Geometry: final body of the model. Coordinates: model frame, mm. Face numbers are marked on the shaded views. Give positions to 0.01 mm unless a question says otherwise; leave off trailing zeros. Order: outer loops, then holes, each group sorted by start corner. A loop starts at its lowest first (then second) coordinate and runs counter-clockwise, first axis right, second up. Notation, with made-up numbers: (81.25, 1.25) - (132.25, 1.25) arc R33 cw to (132.25, 31.25) - close; hole circle Ø1 at (76.5, -34). An arc over 180 degrees is marked (long way). One line per item, written item: value.
```python
from build123d import *

# Parameters (mm, degrees)
SKETCH1_R                 = 3
BOSS_EXTRUDE1_DEPTH       = 24
CHAMFER1_SIZE             = 1
M4X0_7_TAPPED_HOLE1_D     = 3.3
M4X0_7_TAPPED_HOLE1_DEPTH = 6
M4X0_7_TAPPED_HOLE1_TIP   = 0.991420021


with BuildPart() as part:
    # Sketch1 → Boss-Extrude1 (new body)
    with BuildSketch(Plane(origin=(0, 0, 0), x_dir=(1, 0, 0), z_dir=(0, 1, 0))):
        with Locations(Location((0, 0, 0), (0, 0, 270))):
            Circle(SKETCH1_R)
    extrude(amount=BOSS_EXTRUDE1_DEPTH)

    # Chamfer1
    chamfer1_edges = [part.edges().sort_by_distance(p)[0] for p in [
        (0, 24, -3),
    ]]
    chamfer(chamfer1_edges, length=CHAMFER1_SIZE)

    # M4x0.7 Tapped Hole1
    with Locations(Plane.XZ):
        with Locations((0, 0)):
            Hole(M4X0_7_TAPPED_HOLE1_D / 2, depth=M4X0_7_TAPPED_HOLE1_DEPTH)
            with Locations((0, 0, -(M4X0_7_TAPPED_HOLE1_DEPTH + M4X0_7_TAPPED_HOLE1_TIP / 2))):  # 118° drill point
                Cone(0, M4X0_7_TAPPED_HOLE1_D / 2, M4X0_7_TAPPED_HOLE1_TIP, mode=Mode.SUBTRACT)


solid = part.part
```
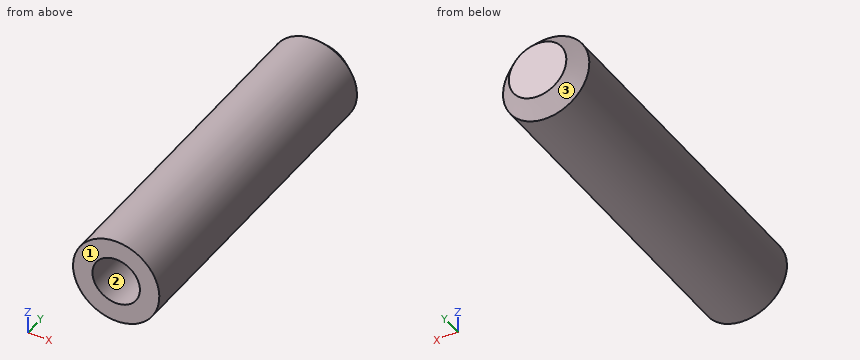
1) Mould query, pull axis X, two halves, no side actions, for the marked faces 1, 2 and 3. Classes: released by +X, released by -X, zero draft, split by the parting line, or undercut.
Answers below:
face 1: zero draft
face 2: undercut
face 3: split by the parting line
2) Section A-A, the plane y = 15. Return loops of the section in (x, z).
Answers below:
outline: circle Ø6 at (0, 0)
3) Material intervals for line 1 along X through (y, z) = (3.05, 0); line 2 along Z through (x, y) = (-0.45, 13.75); line 3 along X through (y, z) = (13, -0.1), sorted ascending.
Answers below:
line 1: -3 to -1.65, 1.65 to 3
line 2: -2.97 to 2.97
line 3: -3 to 3
4) First-contact query: pin 1 (1.5 mm diameter, centred on y = 10, z = -2, fed in from -X). Flat tip, straight axial feed; report the tip coordinate or a pass-through.
Answers below:
pin 1: x = -2.73
